Design review of the part built by this model. Coordinates are the model's own, in mm. Face numbers are marked on the shaded views. A direction names the side the tool comes from. Round coordinates to 2 decimals unless told otherwise and drop trailing zeros. Write each loop counter-clockwise with the first axis right and the second up, starting at its lowest first coordinate (ties: lowest second). Pieces come first, ordered by that corner, then holes. Notation, with made-up numbers: M 48,46 L 68,46 A27 ccw 68,76 Z; hole C 16,-4 d2. An arc over 180 degrees is marked long. Use CSV: the item, a comma, the result in double quotes.
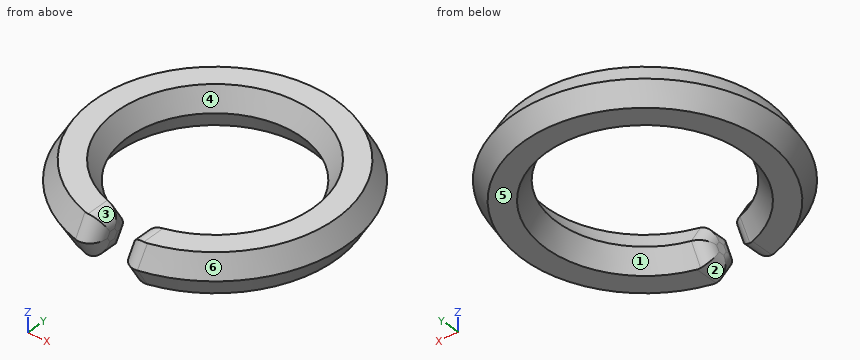
from build123d import *

# Parameters (mm, degrees)
F2_W     = 4.604009
F2_H     = 13.256372
F3_DEPTH = 12.7
F4_R     = 2.54


with BuildPart() as f1:
    # F0 (on Front) → F1 (revolve)
    with BuildSketch(Plane.XZ):
        Polygon((-20.773262, -3.358084), (-16.895681, -3.358084), (-14.95689, 0), (-16.895681, 3.358084), (-20.773262, 3.358084), (-22.712053, 0), align=None)
    revolve(axis=Axis((0, 0, 8.760218), (0, 0, -1)))

    # F2 (on Top) → F3 (cut, symmetric)
    with BuildSketch(Plane.XY):
        with Locations((-0.165461, -17.94427)):
            Rectangle(F2_W, F2_H)
    extrude(amount=F3_DEPTH, both=True, mode=Mode.SUBTRACT)

    # F4
    f4_edges = [f1.edges().sort_by_distance(p)[0] for p in [
        (2.136543, -18.711573, -3.358084),
        (2.136543, -21.637376, -1.679134),
        (2.136543, -21.637376, 1.679134),
        (2.136543, -18.711573, 3.358084),
        (2.136543, -15.782185, 1.678804),
        (2.136543, -15.782185, -1.678804),
        (-2.467466, -18.670366, -3.358084),
        (-2.467466, -15.733794, -1.678721),
        (-2.467466, -15.733794, 1.678721),
        (-2.467466, -18.670366, 3.358084),
        (-2.467466, -21.602122, 1.679166),
        (-2.467466, -21.602122, -1.679166),
    ]]
    fillet(f4_edges, radius=F4_R)


solid = f1.part
1) Add section A-A on y = 0. Write out the cut boundary in (x, z), then the cut area to 3 significant figures.
Answers:
outline,"M -22.71,0 L -20.77,-3.36 L -16.9,-3.36 L -14.96,0 L -16.9,3.36 L -20.77,3.36 Z; M 14.96,0 L 16.9,-3.36 L 20.77,-3.36 L 22.71,0 L 20.77,3.36 L 16.9,3.36 Z"
area,"78.1 mm²"
2) The part is to be moulded in two halves that separate along Y. For the marked faces 4, 5 and 6, say which applies: released by +Y, released by -Y, zero draft, split by the parting line, or undercut.
Answers:
face 4,"undercut"
face 5,"zero draft"
face 6,"split by the parting line"
3) Add section B-B on x = 0. Write out the cut boundary in (y, z), then the cut area to 3 significant figures.
Answers:
outline,"M 14.96,0 L 16.9,-3.36 L 20.77,-3.36 L 22.71,0 L 20.77,3.36 L 16.9,3.36 Z"
area,"39.1 mm²"
4) For pin 1 Ø1.3 at (y, z) = (-18, -0.5) entering from +X; pin 2 Ø1.8 at (y, z) = (-18.5, -0.5) entering from -X; pin 3 Ø1 at (x, z) = (4.5, -0.5) entering from +Y, all flat-tipped, find the tip position at first contact; note any pin that passes through.
Answers:
pin 1,"x = 14.4"
pin 2,"x = -14.17"
pin 3,"y = 22.28"
5) Wall thickness on line 1 along Y through (x, z) = (9.5, 1.75); line 2 along Y through (x, z) = (6.5, 0.5); line 3 along X through (y, z) = (7.5, 1.5): over which ranges is each line inside the solid? List them lowest first. Write a range as [from, to].
Answers:
line 1,"[-19.51, -12.83], [12.83, 19.51]"
line 2,"[-21.46, -13.79], [13.79, 21.46]"
line 3,"[-20.52, -13.93], [13.93, 20.52]"
6) Machinability: for the marked faces 1, 2 and 3, which of the approach directions +Z, -Z, +X, -X, +Y, -Y give a long, thin tool a straight path to every point of the face, cutting with its end or side? Answer none if there is none.
Answers:
face 1,"-Z"
face 2,"-Z, -Y"
face 3,"+Z, -Y"
